Design review of the part shown in the three views and the two pictorial views. Dimensions are in mm from the part's minimum x, y and z. Round coordinates to 2 decimals unless told otherwise and drop trailing zeros. Order: outer loops, then holes, each group sorted by start corner. A loop starts at its lowest first (then second) coordinate and runs counter-clockwise, first axis right, second up.
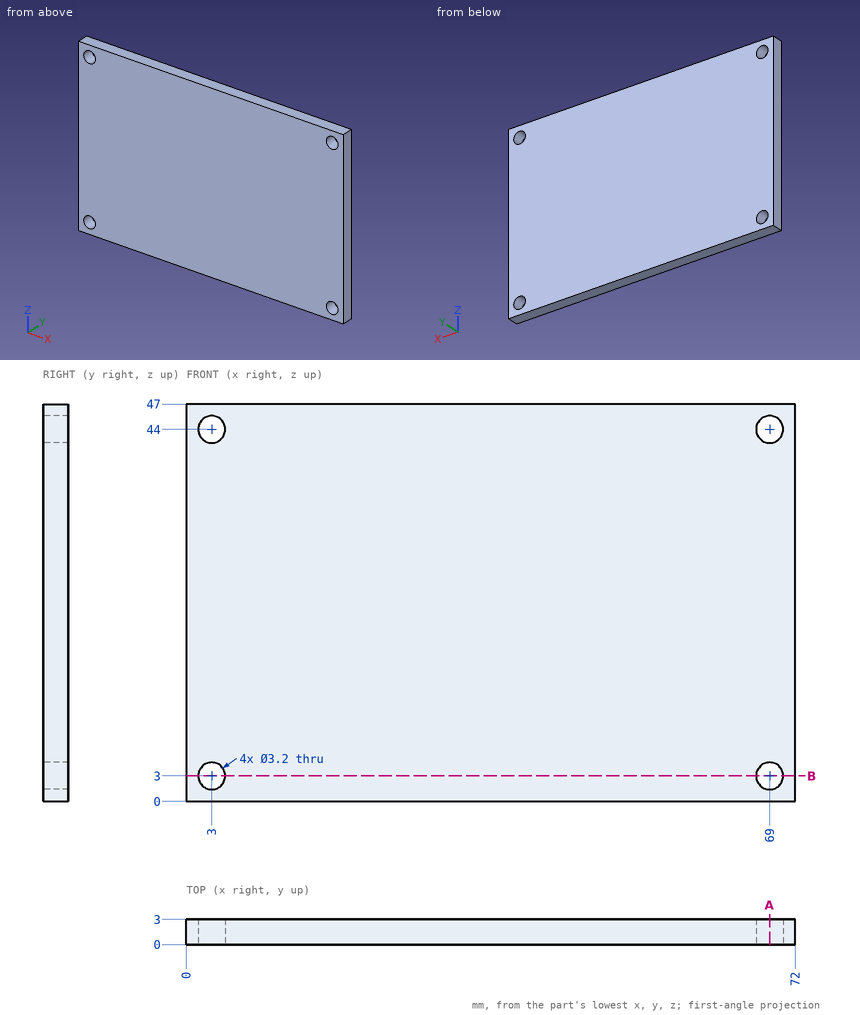
(1) Clearance check with a flat-ended pin moving along its axis: P1, Ø5, axis at x = 3, z = 44, coming from the +Y side. State where the tip first meets the part, or that it passes through.
(2) Add section A-A on x = 69. Give the boundary of the cut face in (y, z).
(3) Add section B-B on z = 3. Give the boundary of the cut face in (x, y), plus the area to 3 significant figures.
(4) Wall thickness on L1, parallel to Z at x = 3, y = 0.95; L2, parallel to X at y = 1.7, z = 44: over which ranges is each line inside the solid? List them lowest first.
Here are the results:
1. P1: stops at y = 3
2. outline: (0, 0) - (3, 0) - (3, 1.4) - (0, 1.4) - close; (0, 4.6) - (3, 4.6) - (3, 42.4) - (0, 42.4) - close; (0, 45.6) - (3, 45.6) - (3, 47) - (0, 47) - close
3. outline: (0, 0) - (1.4, 0) - (1.4, 3) - (0, 3) - close; (4.6, 0) - (67.4, 0) - (67.4, 3) - (4.6, 3) - close; (70.6, 0) - (72, 0) - (72, 3) - (70.6, 3) - close
3. area: 197 mm2
4. L1: z = 0 to 1.4, 4.6 to 42.4, 45.6 to 47
4. L2: x = 0 to 1.4, 4.6 to 67.4, 70.6 to 72
